Here's how the part is built. I have some questions about the finished solid (model axes, mm). A direction names the side the tool comes from. Round coordinates to 2 decimals unless told otherwise and drop trailing zeros. Loops run counter-clockwise (first coordinate to the right, second up) from the corner with the lowest first, then second, coordinate; pieces in that order, holes last. Notation, with made-up numbers: M -21.75,70.25 L -10.75,70.25 A28 ccw -10.75,96.25 Z; hole C 66,47.25 d10. An arc over 180 degrees is marked long. Answer as CSV lines item,"result".
```python
from build123d import *

# Parameters (mm, degrees)
F3_D      = 3.25
F6_R      = 1.625
F8_R      = 1.625
F9_DEPTH  = 15
F11_DEPTH = 15
F13_DEPTH = 20


with BuildPart() as f1:
    # F0 (on Front) → F1 (revolve)
    with BuildSketch(Plane.XZ):
        Polygon((0, 10), (0, 0), (2.75, 0), (2.25, 10), align=None)
    revolve(axis=Axis((0, 0, 5), (0, 0, -1)))

    # F3 (through all)
    with Locations(Plane.XY.offset(10)):
        with Locations((0, 0)):
            Hole(F3_D / 2)


with BuildPart() as f4_1:
    # F4: copy of F1
    add(f1.part.moved(Location((10, 0, 0))))


with BuildPart() as f7:
    # F7: sweep along a path in F5
    with BuildLine(Plane.XZ) as f7_path:
        ThreePointArc((10, 0), (7.0710678119, -7.0710678119), (0, -10))
    # F6 (on face) → F7 (sweep)
    with BuildSketch(Plane(origin=(0, 0, 0), x_dir=(1, 0, 0), z_dir=(0, 0, -1))):
        with Locations((10, 0)):
            Circle(F6_R)
    sweep(path=f7_path.line)

    # F8 (on face) → F9 (join)
    with BuildSketch(Plane(origin=(0, 0, 0), x_dir=(1, 0, 0), z_dir=(0, 0, -1))):
        Circle(F8_R)
    extrude(amount=F9_DEPTH)


with BuildPart() as f11:
    # F10 (on Top) → F11 (new body)
    with BuildSketch(Plane.XY):
        with BuildLine():
            Line((10, 2.75), (0, 2.75))
            ThreePointArc((0, 2.75), (-2.75, 0), (0, -2.75))
            Line((0, -2.75), (10, -2.75))
            ThreePointArc((10, -2.75), (12.75, 0), (10, 2.75))
        make_face()
    extrude(amount=-F11_DEPTH)

    # F12: cut F7
    add(f7.part, mode=Mode.SUBTRACT)


with BuildPart() as f1_1:
    add(f1.part)

    # F13 (add): a face of the model
    f13_faces = [f11.part.faces().sort_by_distance(p)[0] for p in [
        (5.5886652474, 0, -15),
    ]]

    add(f4_1.part)  # F13 merges F4_1

    add(f11.part)  # F13 merges F11
    extrude(f13_faces, amount=F13_DEPTH)


solid = f1_1.part
```
1. Which directions (+Z, -Z, +X, -X, +Y, -Y) give clear straight access to the entire face, cutting with the end or side of a thin tool? Please do faces 1 (the flat face through (5, 0, 0)), 2 (the flat face through (5, 0, -35)).
Evaluation:
face 1,"+Z"
face 2,"-Z, +X, -X, +Y, -Y"
2. I want a section at B-B, the plane y = 0. Please give me the cut outline in (x, z) (3 decimals), and give its area (3 significant figures).
Evaluation:
outline,"M -2.75,-35 L -1.625,-35 L -1.625,10 L -2.25,10 L -2.75,0 Z; M 1.625,-35 L 12.75,-35 L 12.75,0 L 12.25,10 L 11.625,10 L 11.625,0 A11.625 cw 1.625,-11.511 Z; M 1.625,-8.216 A8.375 ccw 8.375,0 L 8.375,10 L 7.75,10 L 7.25,0 L 2.75,0 L 2.25,10 L 1.625,10 Z"
area,"418 mm²"
3. I want a section at A-A, the plane z = -15.5. Please give me the cut outline in (x, y) (3 decimals).
Evaluation:
outline,"M 0,-2.75 L 10,-2.75 A2.75 ccw 10,2.75 L 0,2.75 A2.75 ccw Z; hole C 0,0 d3.25"
4. For P1, Ø1.9, axis at x = 0, y = 0, coming from the +Z side, with a flat end and sliding along its axis, tell me the tip position at first contact or that it passes through.
Evaluation:
P1,"passes through"
5. I want a section at C-C, the plane z = -6.5. Count the separate pieces of the cut face and the enclosed holes in it, and give its area (3 significant figures).
Evaluation:
separate pieces,"1"
enclosed holes,"2"
area,"59.4 mm²"
6. We'd pull the mould along X, two halves only. Please class faces 3 (the cylindrical face through (-2.75, 0.06, -17.26)), 4 (the cylindrical face through (11.623, 0.071, 4.93)), 5 (the flat face through (12, 0, 10)), 6 (the cylindrical face through (12.75, -0.06, -17.26)): pulls with the +X half, pulls with the -X half, needs draft (parallel to the pull), parting line crosses it, or undercut.
Evaluation:
face 3,"pulls with the -X half"
face 4,"undercut"
face 5,"needs draft"
face 6,"pulls with the +X half"
7. If I drill on line 1 (X direction, y = 0, z = 7) (3 decimals); line 2 (X direction, y = -0.6, z = -7); line 3 (X direction, y = 0, z = -5.75) (3 decimals), over which ranges is the centre line in solid material (lowest first)? Write a range as [from, to].
Evaluation:
line 1,"x = [-2.4, -1.625], [1.625, 2.4], [7.6, 8.375], [11.625, 12.4]"
line 2,"x = [-2.68, -1.51], [1.51, 4.8], [9.14, 12.68]"
line 3,"x = [-2.75, -1.625], [1.625, 6.089], [10.103, 12.75]"
